from build123d import *

# Parameters (mm, degrees)
BOSS_EXTRUDE1_DEPTH = 3


with BuildPart() as part:
    # Sketch1 → Boss-Extrude1 (new body)
    with BuildSketch(Plane.XY):
        with BuildLine():
            Line((0, 0), (-20, 0))
            Line((-20, 0), (-20, -3))
            Line((-20, -3), (-50, -3))
            Line((-50, -3), (-50, 0))
            Line((-50, 0), (-70, 0))
            Line((-70, 0), (-70, 10))
            Line((-70, 10), (-60, 10))
            ThreePointArc((-60, 10), (-35, 4.543560573), (-10, 10))
            ThreePointArc((-10, 10), (-4.101453402, 14.101453402), (0, 20))
            Line((0, 20), (0, 0))
        make_face()
    extrude(amount=BOSS_EXTRUDE1_DEPTH)


solid = part.part
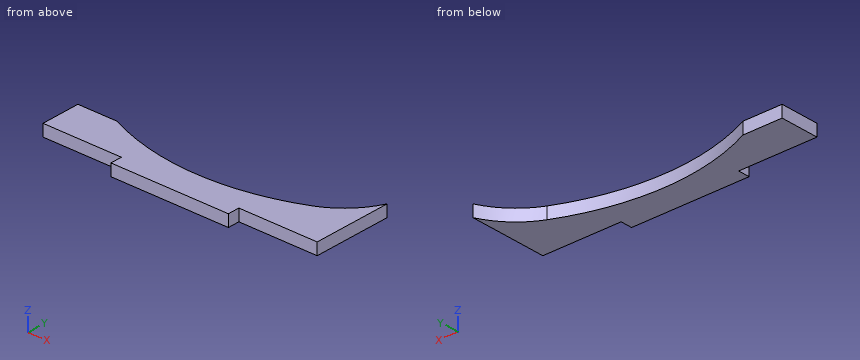
The listing builds one solid part. Answer for the finished solid, in the listing's coordinates (mm). Give positions to 0.01 mm unless a question says otherwise; leave off trailing zeros. Loops run counter-clockwise (first coordinate to the right, second up) from the corner with the lowest first, then second, coordinate; pieces in that order, holes last.
Item 1: A cutting plane is placed at C-C (x = -65). Give the vertices of the cut face in (y, z), then the cut area to 3 significant figures.
Derived:
outline: (0, 0) - (10, 0) - (10, 3) - (0, 3) - close
area: 30.0 mm2
Item 2: A cutting plane is placed at A-A (y = 5.75). Give the vertices of the cut face in (x, z), then the cut area to 3 significant figures.
Derived:
outline: (-70, 0) - (-46.97, 0) - (-46.97, 3) - (-70, 3) - close; (-23.03, 0) - (0, 0) - (0, 3) - (-23.03, 3) - close
area: 138 mm2
Item 3: Each of these flat-tipped pins is pushed along its axis until it touches: pin 1 Ø0.9 at (y, z) = (-2, 1) entering from -X; pin 2 Ø1.5 at (y, z) = (-2, 2) entering from +X; pin 3 Ø1.5 at (x, z) = (-66.5, 1.5) entering from +Y. Where does it stop, or does it pass through?
Derived:
pin 1: stops at x = -50
pin 2: stops at x = -20
pin 3: stops at y = 10
Item 4: A cutting plane is placed at D-D (y = 9.25). Give the vertices of the cut face in (x, z), then the cut area to 3 significant figures.
Derived:
outline: (-70, 0) - (-58.29, 0) - (-58.29, 3) - (-70, 3) - close; (-11.71, 0) - (0, 0) - (0, 3) - (-11.71, 3) - close
area: 70.2 mm2
Item 5: A cutting plane is placed at B-B (z = 0.45). Give the vertices of the cut face in (x, y).
Derived:
outline: (-70, 0) - (-50, 0) - (-50, -3) - (-20, -3) - (-20, 0) - (0, 0) - (0, 20) arc R20.31 cw to (-10, 10) arc R60 cw to (-60, 10) - (-70, 10) - close
Item 6: Find the intervals of material crossed by line 1 along Y through (x, z) = (-21, 1.95); line 2 along Y through (x, z) = (-42, 1.45); line 3 along X through (y, z) = (15, 2.55), in increasing order.
Derived:
line 1: y = -3 to 6.2
line 2: y = -3 to 4.95
line 3: x = -3.26 to 0
